Source: CAD feature listing. Evaluate the final solid. Frame: model axes, mm. A direction names the side the tool comes from. Give positions to 0.01 mm unless a question says otherwise; leave off trailing zeros. Loops run counter-clockwise (first coordinate to the right, second up) from the corner with the lowest first, then second, coordinate; pieces in that order, holes last. Notation, with made-up numbers: M -16,50 L 35,50 A27 ccw 35,67 Z; hole C 33,-11.75 d6. An arc over 180 degrees is marked long. Answer in a Markdown table with one row per item.
```python
from build123d import *

# Parameters (mm, degrees)
SKETCH1_R           = 57.5
SKETCH1_R_2         = 39
SKETCH1_R_3         = 2
SKETCH1_R_4         = 2.5
BOSS_EXTRUDE1_DEPTH = 10
SKETCH2_R           = 2.5
CUT_EXTRUDE1_DEPTH  = 10
SKETCH4_R           = 5
SKETCH4_R_2         = 2.5
BOSS_EXTRUDE3_DEPTH = 0.4


with BuildPart() as part:
    # Sketch1 → Boss-Extrude1 (new body)
    with BuildSketch(Plane(origin=(0, 0, 0), x_dir=(1, 0, 0), z_dir=(0, 1, 0))):
        with Locations(Location((0, 0, 0), (0, 0, 270))):
            Circle(SKETCH1_R)
        with Locations(Location((0, 0, 0), (0, 0, 270))):
            Circle(SKETCH1_R_2, mode=Mode.SUBTRACT)
        with Locations(Location((0, 54, 0), (0, 0, 270))):
            Circle(SKETCH1_R_3, mode=Mode.SUBTRACT)
        with Locations(Location((27, 46.765371804, 0), (0, 0, 270))):
            Circle(SKETCH1_R_3, mode=Mode.SUBTRACT)
        with Locations(Location((46.765371804, 27, 0), (0, 0, 270))):
            Circle(SKETCH1_R_3, mode=Mode.SUBTRACT)
        with Locations(Location((54, 0, 0), (0, 0, 270))):
            Circle(SKETCH1_R_3, mode=Mode.SUBTRACT)
        with Locations(Location((46.765371804, -27, 0), (0, 0, 270))):
            Circle(SKETCH1_R_3, mode=Mode.SUBTRACT)
        with Locations(Location((27, -46.765371804, 0), (0, 0, 270))):
            Circle(SKETCH1_R_3, mode=Mode.SUBTRACT)
        with Locations(Location((0, -54, 0), (0, 0, 270))):
            Circle(SKETCH1_R_3, mode=Mode.SUBTRACT)
        with Locations(Location((-27, -46.765371804, 0), (0, 0, 270))):
            Circle(SKETCH1_R_3, mode=Mode.SUBTRACT)
        with Locations(Location((-46.765371804, -27, 0), (0, 0, 270))):
            Circle(SKETCH1_R_3, mode=Mode.SUBTRACT)
        with Locations(Location((-54, 0, 0), (0, 0, 270))):
            Circle(SKETCH1_R_3, mode=Mode.SUBTRACT)
        with Locations(Location((-46.765371804, 27, 0), (0, 0, 270))):
            Circle(SKETCH1_R_3, mode=Mode.SUBTRACT)
        with Locations(Location((-27, 46.765371804, 0), (0, 0, 270))):
            Circle(SKETCH1_R_3, mode=Mode.SUBTRACT)
        with Locations(Location((13.587999868, 50.71110588, 0), (0, 0, 270))):
            Circle(SKETCH1_R_4, mode=Mode.SUBTRACT)
        with Locations(Location((37.123106012, 37.123106012, 0), (0, 0, 270))):
            Circle(SKETCH1_R_4, mode=Mode.SUBTRACT)
        with Locations(Location((50.71110588, 13.587999868, 0), (0, 0, 270))):
            Circle(SKETCH1_R_4, mode=Mode.SUBTRACT)
        with Locations(Location((50.71110588, -13.587999868, 0), (0, 0, 270))):
            Circle(SKETCH1_R_4, mode=Mode.SUBTRACT)
        with Locations(Location((37.123106012, -37.123106012, 0), (0, 0, 270))):
            Circle(SKETCH1_R_4, mode=Mode.SUBTRACT)
        with Locations(Location((13.587999868, -50.71110588, 0), (0, 0, 270))):
            Circle(SKETCH1_R_4, mode=Mode.SUBTRACT)
        with Locations(Location((-13.587999868, -50.71110588, 0), (0, 0, 270))):
            Circle(SKETCH1_R_4, mode=Mode.SUBTRACT)
        with Locations(Location((-37.123106012, -37.123106012, 0), (0, 0, 270))):
            Circle(SKETCH1_R_4, mode=Mode.SUBTRACT)
        with Locations(Location((-50.71110588, -13.587999868, 0), (0, 0, 270))):
            Circle(SKETCH1_R_4, mode=Mode.SUBTRACT)
        with Locations(Location((-50.71110588, 13.587999868, 0), (0, 0, 270))):
            Circle(SKETCH1_R_4, mode=Mode.SUBTRACT)
        with Locations(Location((-37.123106012, 37.123106012, 0), (0, 0, 270))):
            Circle(SKETCH1_R_4, mode=Mode.SUBTRACT)
        with Locations(Location((-13.587999868, 50.71110588, 0), (0, 0, 270))):
            Circle(SKETCH1_R_4, mode=Mode.SUBTRACT)
    extrude(amount=BOSS_EXTRUDE1_DEPTH)

    # Sketch2 → Cut-Extrude1 (cut)
    with BuildSketch(Plane(origin=(0, 10, 0), x_dir=(1, 0, 0), z_dir=(0, 1, 0))):
        with Locations(Location((0, 45, 0), (0, 0, 270))):
            Circle(SKETCH2_R)
        with Locations(Location((24.328836786, 37.856408977, 0), (0, 0, 270))):
            Circle(SKETCH2_R)
        with Locations(Location((40.933439791, 18.693675585, 0), (0, 0, 270))):
            Circle(SKETCH2_R)
        with Locations(Location((44.541964885, -6.404167722, 0), (0, 0, 270))):
            Circle(SKETCH2_R)
        with Locations(Location((34.008730846, -29.468733028, 0), (0, 0, 270))):
            Circle(SKETCH2_R)
        with Locations(Location((12.677965058, -43.177183813, 0), (0, 0, 270))):
            Circle(SKETCH2_R)
        with Locations(Location((-12.677965058, -43.177183813, 0), (0, 0, 270))):
            Circle(SKETCH2_R)
        with Locations(Location((-34.008730846, -29.468733028, 0), (0, 0, 270))):
            Circle(SKETCH2_R)
        with Locations(Location((-44.541964885, -6.404167722, 0), (0, 0, 270))):
            Circle(SKETCH2_R)
        with Locations(Location((-40.933439791, 18.693675585, 0), (0, 0, 270))):
            Circle(SKETCH2_R)
        with Locations(Location((-24.328836786, 37.856408977, 0), (0, 0, 270))):
            Circle(SKETCH2_R)
    extrude(amount=-CUT_EXTRUDE1_DEPTH, mode=Mode.SUBTRACT)

    # Sketch4 → Boss-Extrude3 (add)
    # profile 1 of 11: a face of its own
    with BuildSketch(Plane(origin=(0, 0, 0), x_dir=(1, 0, 0), z_dir=(0, 1, 0))):
        with Locations(Location((0, 45, 0), (0, 0, 270))):
            Circle(SKETCH4_R)
        with Locations(Location((0, 45, 0), (0, 0, 270))):
            Circle(SKETCH4_R_2, mode=Mode.SUBTRACT)
    # profile 2 of 11: a face of its own
    with BuildSketch(Plane(origin=(0, 0, 0), x_dir=(1, 0, 0), z_dir=(0, 1, 0))):
        with Locations(Location((24.328836786, 37.856408977, 0), (0, 0, 270))):
            Circle(SKETCH4_R)
        with Locations(Location((24.328836786, 37.856408977, 0), (0, 0, 270))):
            Circle(SKETCH4_R_2, mode=Mode.SUBTRACT)
    # profile 3 of 11: a face of its own
    with BuildSketch(Plane(origin=(0, 0, 0), x_dir=(1, 0, 0), z_dir=(0, 1, 0))):
        with Locations(Location((40.933439791, 18.693675585, 0), (0, 0, 270))):
            Circle(SKETCH4_R)
        with Locations(Location((40.933439791, 18.693675585, 0), (0, 0, 270))):
            Circle(SKETCH4_R_2, mode=Mode.SUBTRACT)
    # profile 4 of 11: a face of its own
    with BuildSketch(Plane(origin=(0, 0, 0), x_dir=(1, 0, 0), z_dir=(0, 1, 0))):
        with Locations(Location((44.541964885, -6.404167722, 0), (0, 0, 270))):
            Circle(SKETCH4_R)
        with Locations(Location((44.541964885, -6.404167722, 0), (0, 0, 270))):
            Circle(SKETCH4_R_2, mode=Mode.SUBTRACT)
    # profile 5 of 11: a face of its own
    with BuildSketch(Plane(origin=(0, 0, 0), x_dir=(1, 0, 0), z_dir=(0, 1, 0))):
        with Locations(Location((34.008730846, -29.468733028, 0), (0, 0, 270))):
            Circle(SKETCH4_R)
        with Locations(Location((34.008730846, -29.468733028, 0), (0, 0, 270))):
            Circle(SKETCH4_R_2, mode=Mode.SUBTRACT)
    # profile 6 of 11: a face of its own
    with BuildSketch(Plane(origin=(0, 0, 0), x_dir=(1, 0, 0), z_dir=(0, 1, 0))):
        with Locations(Location((12.677965058, -43.177183813, 0), (0, 0, 270))):
            Circle(SKETCH4_R)
        with Locations(Location((12.677965058, -43.177183813, 0), (0, 0, 270))):
            Circle(SKETCH4_R_2, mode=Mode.SUBTRACT)
    # profile 7 of 11: a face of its own
    with BuildSketch(Plane(origin=(0, 0, 0), x_dir=(1, 0, 0), z_dir=(0, 1, 0))):
        with Locations(Location((-12.677965058, -43.177183813, 0), (0, 0, 270))):
            Circle(SKETCH4_R)
        with Locations(Location((-12.677965058, -43.177183813, 0), (0, 0, 270))):
            Circle(SKETCH4_R_2, mode=Mode.SUBTRACT)
    # profile 8 of 11: a face of its own
    with BuildSketch(Plane(origin=(0, 0, 0), x_dir=(1, 0, 0), z_dir=(0, 1, 0))):
        with Locations(Location((-34.008730846, -29.468733028, 0), (0, 0, 270))):
            Circle(SKETCH4_R)
        with Locations(Location((-34.008730846, -29.468733028, 0), (0, 0, 270))):
            Circle(SKETCH4_R_2, mode=Mode.SUBTRACT)
    # profile 9 of 11: a face of its own
    with BuildSketch(Plane(origin=(0, 0, 0), x_dir=(1, 0, 0), z_dir=(0, 1, 0))):
        with Locations(Location((-44.541964885, -6.404167722, 0), (0, 0, 270))):
            Circle(SKETCH4_R)
        with Locations(Location((-44.541964885, -6.404167722, 0), (0, 0, 270))):
            Circle(SKETCH4_R_2, mode=Mode.SUBTRACT)
    # profile 10 of 11: a face of its own
    with BuildSketch(Plane(origin=(0, 0, 0), x_dir=(1, 0, 0), z_dir=(0, 1, 0))):
        with Locations(Location((-40.933439791, 18.693675585, 0), (0, 0, 270))):
            Circle(SKETCH4_R)
        with Locations(Location((-40.933439791, 18.693675585, 0), (0, 0, 270))):
            Circle(SKETCH4_R_2, mode=Mode.SUBTRACT)
    # profile 11 of 11: a face of its own
    with BuildSketch(Plane(origin=(0, 0, 0), x_dir=(1, 0, 0), z_dir=(0, 1, 0))):
        with Locations(Location((-24.328836786, 37.856408977, 0), (0, 0, 270))):
            Circle(SKETCH4_R)
        with Locations(Location((-24.328836786, 37.856408977, 0), (0, 0, 270))):
            Circle(SKETCH4_R_2, mode=Mode.SUBTRACT)
    extrude(amount=-BOSS_EXTRUDE3_DEPTH)


solid = part.part
```
1) Pull-direction query (X, two-part tool) for faces 1 (the cylindrical face through (44.99, 4.93, -26.08)), 2 (the cylindrical face through (52.401, 4.93, 11.745)), 3 (the flat face through (47, -0.4, 5)); classes: released by +X, released by -X, zero draft, split by the parting line, or undercut.
Reply:
| item | result |
|---|---|
| face 1 | undercut |
| face 2 | undercut |
| face 3 | zero draft |
2) Set-up query: faces 4 (the cylindrical face through (-28.765, -0.197, -35.549)), 5 (the cylindrical face through (0, 5, 52)). Return all of +Z, -Z, +X, -X, +Y, -Y with unobstructed straight access to the full face (end or side cutting, diameter ignored); none if empty.
Reply:
| item | result |
|---|---|
| face 4 | -Y |
| face 5 | +Y, -Y |
3) Section C-C, the plane z = 19. Return loops of the section in (x, y).
Reply:
| item | result |
|---|---|
| outline | M -54.27,0 L -34.06,0 L -34.06,10 L -54.27,10 Z; M 34.06,0 L 54.27,0 L 54.27,10 L 34.06,10 Z |
4) Section B-B, the plane z = 42.5. Return loops of the section in (x, y).
Reply:
| item | result |
|---|---|
| outline | M -38.73,0 L -17.63,0 L -17.63,-0.4 L -15.08,-0.4 L -15.08,10 L -38.73,10 Z; M -10.27,-0.4 L -7.72,-0.4 L -7.72,0 L 7.72,0 L 7.72,-0.4 L 10.27,-0.4 L 10.27,10 L -10.27,10 Z; M 15.08,-0.4 L 17.63,-0.4 L 17.63,0 L 38.73,0 L 38.73,10 L 15.08,10 Z |
5) Material intervals for L1, parallel to Z at x = 48.5, y = 1; L2, parallel to Z at x = -14.5, y = 1.25; L3, parallel to X at y = 6.75, z = -40, sorted ascending.
Reply:
| item | result |
|---|---|
| L1 | z = -30.89 to -28, -26 to -14.75, -12.42 to 12.42, 14.75 to 26, 28 to 30.89 |
| L2 | z = -55.64 to -53.04, -48.38 to -36.2, 36.2 to 41.47, 44.89 to 48.38, 53.04 to 55.64 |
| L3 | x = -41.31 to -25.62, -23.04 to 23.04, 25.62 to 41.31 |
6) Pin query (flat end, axial travel): pin 1 Ø1.5 at (y, z) = (1, 27.5) entering from -X; pin 2 Ø5 at (x, y) = (34, 7.5) entering from -Z; pin 3 Ø3 at (y, z) = (1.5, 26) entering from +X. Return the tip coordinate at first contact, or that it passes through.
Reply:
| item | result |
|---|---|
| pin 1 | stops at x = -50.9 |
| pin 2 | stops at z = -48.1 |
| pin 3 | stops at x = 52.02 |
7) Section A-A, the plane x = 0. Return loops of the section in (y, z), then the cut area to 3 significant figures.
Reply:
| item | result |
|---|---|
| outline | M -0.4,-50 L 0,-50 L 0,-52 L 10,-52 L 10,-47.5 L -0.4,-47.5 Z; M -0.4,-42.5 L 10,-42.5 L 10,-39 L 0,-39 L 0,-40 L -0.4,-40 Z; M 0,-57.5 L 10,-57.5 L 10,-56 L 0,-56 Z; M 0,39 L 10,39 L 10,52 L 0,52 Z; M 0,56 L 10,56 L 10,57.5 L 0,57.5 Z |
| area | 242 mm² |
